Can you work these out from the model? Positions are in its coordinate system, mm. A direction names the side the tool comes from. Give positions to 0.01 mm unless a question says otherwise; leave off trailing zeros. Loops run counter-clockwise (first coordinate to the right, second up) from the corner with the lowest first, then second, coordinate; pieces in that order, holes last. Notation, with made-up numbers: M 5.25,52 L 22.25,52 A35 ccw 22.25,86 Z; hole C -32.5,21 d1. An arc over 180 degrees is marked long. Answer as a JSON object with one key per item and string values.
```python
from build123d import *

# Parameters (mm, degrees)
BOSS_EXTRUDE1_DEPTH  = 49
SKETCH2_R            = 2.5
CUT_EXTRUDE1_DEPTH   = 8.5
SKETCH4_W            = 79
SKETCH4_H            = 39.5
BOSS_EXTRUDE2_DEPTH  = 6
BOSS_EXTRUDE3_DEPTH  = 4
SKETCH5_R            = 2
CUT_EXTRUDE3_DEPTH   = 10
BOSS_EXTRUDE4_DEPTH  = 4
SKETCH8_R            = 1.5
CUT_EXTRUDE4_DEPTH   = 8
FILLET1_R            = 6
FILLET2_R            = 5
CUT_EXTRUDE5_DEPTH   = 3
CUT_EXTRUDE6_DEPTH   = 50
FILLET3_R            = 4
CUT_EXTRUDE7_DEPTH   = 3
LPATTERN1_COUNT      = 2
LPATTERN1_PITCH      = 67
LPATTERN1_COUNT_DIR2 = 2
LPATTERN1_PITCH_DIR2 = 27.5


with BuildPart() as part:
    # Sketch1 → Boss-Extrude1 (new body)
    with BuildSketch(Plane.XY):
        Polygon((4, 7.5), (4, 19.5), (0, 19.5), (0, 0), (55, 0), (55, 7.5), align=None)
    extrude(amount=BOSS_EXTRUDE1_DEPTH)

    # Sketch2 → Cut-Extrude1 (cut, through all)
    with BuildSketch(Plane(origin=(0, 7.5, 0), x_dir=(1, 0, 0), z_dir=(0, 1, 0))):
        with Locations(Location((12, -12.5, 0), (0, 0, 270))):  # turned: the seam where the file's is
            Circle(SKETCH2_R)
        with Locations(Location((43, -12.5, 0), (0, 0, 270))):  # turned: the seam where the file's is
            Circle(SKETCH2_R)
        with Locations(Location((12, -43.5, 0), (0, 0, 270))):  # turned: the seam where the file's is
            Circle(SKETCH2_R)
        with Locations(Location((43, -43.5, 0), (0, 0, 270))):  # turned: the seam where the file's is
            Circle(SKETCH2_R)
        with BuildLine():
            Line((14.460001345, -31.494057109), (19.150704606, -49))
            Line((19.150704606, -49), (35.849295394, -49))
            Line((35.849295394, -49), (40.539998655, -31.494057109))
            ThreePointArc((40.539998655, -31.494057109), (27.5, -14.5), (14.460001345, -31.494057109))
        make_face()
    extrude(amount=-CUT_EXTRUDE1_DEPTH, mode=Mode.SUBTRACT)

    # Sketch4 → Boss-Extrude2 (add)
    with BuildSketch(Plane(origin=(0, 0, 0), x_dir=(-1, 0, 0), z_dir=(0, 0, -1))):
        with Locations((-27.5, -0.25)):
            Rectangle(SKETCH4_W, SKETCH4_H)
    extrude(amount=-BOSS_EXTRUDE2_DEPTH)

    # Sketch6 → Boss-Extrude3 (add)
    with BuildSketch(Plane.ZY):
        Polygon((6, -20), (49, 0), (6, 0), align=None)
    extrude(amount=-BOSS_EXTRUDE3_DEPTH)

    # Sketch5 → Cut-Extrude3 (cut)
    with BuildSketch(Plane(origin=(0, 0, 0), x_dir=(-1, 0, 0), z_dir=(0, 0, -1))):
        with Locations((-61, 13.5)):
            Circle(SKETCH5_R)
        with Locations((-61, -14)):
            Circle(SKETCH5_R)
        with Locations((6, 13.5)):
            Circle(SKETCH5_R)
        with Locations((6, -14)):
            Circle(SKETCH5_R)
    extrude(amount=-CUT_EXTRUDE3_DEPTH, mode=Mode.SUBTRACT)

    # Sketch7 → Boss-Extrude4 (add)
    with BuildSketch(Plane(origin=(55, 0, 0), x_dir=(0, 0, -1), z_dir=(1, 0, 0))):
        Polygon((-49, 7.5), (-6, 19.5), (0, 19.5), (0, -20), (-6, -20), (-49, 0), align=None)
    extrude(amount=-BOSS_EXTRUDE4_DEPTH)

    # Sketch8 → Cut-Extrude4 (cut)
    with BuildSketch(Plane.ZY):
        with Locations(Location((43, 13, 0), (0, 0, 270))):  # turned: the seam where the file's is
            Circle(SKETCH8_R)
        with Locations(Location((43, 3.5, 0), (0, 0, 270))):  # turned: the seam where the file's is
            Circle(SKETCH8_R)
    extrude(amount=-CUT_EXTRUDE4_DEPTH, mode=Mode.SUBTRACT)

    # Fillet1
    fillet1_edges = [part.edges().sort_by_distance(p)[0] for p in [
        (67, 19.5, 3),
        (-12, 19.5, 3),
        (-12, -20, 3),
        (67, -20, 3),
    ]]
    fillet(fillet1_edges, radius=FILLET1_R)

    # Fillet2
    fillet2_edges = [part.edges().sort_by_distance(p)[0] for p in [
        (35.849295394, 3.75, 49),
        (19.150704606, 3.75, 49),
    ]]
    fillet(fillet2_edges, radius=FILLET2_R)

    # Sketch9 → Cut-Extrude5 (cut)
    with BuildSketch(Plane.XY.offset(6)):
        Polygon((-6, 16.790896534), (-8.85, 15.145448267), (-8.85, 11.854551733), (-6, 10.209103466), (-3.15, 11.854551733), (-3.15, 15.145448267), align=None)
        Polygon((-6, -10.709103466), (-8.85, -12.354551733), (-8.85, -15.645448267), (-6, -17.290896534), (-3.15, -15.645448267), (-3.15, -12.354551733), align=None)
        Polygon((61, -10.709103466), (58.15, -12.354551733), (58.15, -15.645448267), (61, -17.290896534), (63.85, -15.645448267), (63.85, -12.354551733), align=None)
        Polygon((61, 10.209103466), (63.85, 11.854551733), (63.85, 15.145448267), (61, 16.790896534), (58.15, 15.145448267), (58.15, 11.854551733), align=None)
    extrude(amount=-CUT_EXTRUDE5_DEPTH, mode=Mode.SUBTRACT)

    # Sketch10 → Cut-Extrude6 (cut, through all)
    with BuildSketch(Plane(origin=(0, 0, 0), x_dir=(-1, 0, 0), z_dir=(0, 0, -1))):
        with BuildLine():
            Line((-61, 19.5), (-61, 26.194717678))
            Line((-61, 26.194717678), (-93.21372943, 26.194717678))
            Line((-93.21372943, 26.194717678), (-93.21372943, -32.483465835))
            Line((-93.21372943, -32.483465835), (20.656804912, -32.483465835))
            Line((20.656804912, -32.483465835), (20.656804912, 27.240467483))
            Line((20.656804912, 27.240467483), (6, 27.240467483))
            Line((6, 27.240467483), (6, 19.5))
            ThreePointArc((6, 19.5), (10.987484336, 16.835416016), (11.545111711, 11.208333333))
            ThreePointArc((11.545111711, 11.208333333), (9.270670267, -0.25), (11.545111711, -11.708333333))
            ThreePointArc((11.545111711, -11.708333333), (10.460015748, -18.013509627), (4.303797468, -19.755249514))
            ThreePointArc((4.303797468, -19.755249514), (-27.5, -15.166177907), (-59.303797468, -19.755249514))
            ThreePointArc((-59.303797468, -19.755249514), (-65.460015748, -18.013509627), (-66.545111711, -11.708333333))
            ThreePointArc((-66.545111711, -11.708333333), (-64.270670267, -0.25), (-66.545111711, 11.208333333))
            ThreePointArc((-66.545111711, 11.208333333), (-65.987484336, 16.835416016), (-61, 19.5))
        make_face()
    extrude(amount=-CUT_EXTRUDE6_DEPTH, mode=Mode.SUBTRACT)

    # Fillet3
    fillet3_edges = [part.edges().sort_by_distance(p)[0] for p in [
        (2, 19.5, 49),
    ]]
    fillet(fillet3_edges, radius=FILLET3_R)

    # Sketch11 → Cut-Extrude7 (cut)
    with BuildSketch(Plane.XY.offset(6)):
        with BuildLine():
            ThreePointArc((-9.35, 15.434123402), (-8.85, 13.5), (-9.35, 11.565876598))
            ThreePointArc((-9.35, 11.565876598), (-7.425, 11.031827599), (-6, 9.631753196))
            ThreePointArc((-6, 9.631753196), (-4.575, 11.031827599), (-2.65, 11.565876598))
            ThreePointArc((-2.65, 11.565876598), (-3.15, 13.5), (-2.65, 15.434123402))
            ThreePointArc((-2.65, 15.434123402), (-4.575, 15.968172401), (-6, 17.368246804))
            ThreePointArc((-6, 17.368246804), (-7.425, 15.968172401), (-9.35, 15.434123402))
        make_face()
    cut_extrude7 = extrude(amount=-CUT_EXTRUDE7_DEPTH, mode=Mode.SUBTRACT)

    # LPattern1: Cut-Extrude7 2 × 2
    with Locations(*[(i * LPATTERN1_PITCH, -j * LPATTERN1_PITCH_DIR2, 0) for i in range(LPATTERN1_COUNT) for j in range(LPATTERN1_COUNT_DIR2) if (i, j) != (0, 0)]):
        add(cut_extrude7, mode=Mode.SUBTRACT)


solid = part.part
```
1) If we mould it in two halves opening along Z, with no side actions, what happens to faces 1 (the flat face through (28, 0, 0)), 2 (the cylindrical face through (1.972, 13.325, 41.536)), 3 (the flat face through (39.017, 3.802, 37.178)), 4 (the cylindrical face through (62.474, 14.852, 1.479))? For each: +Z half, -Z half, draft (parallel to the pull), parting line (faces both ways), or undercut.
Answer list:
{"face 1": "-Z half", "face 2": "undercut", "face 3": "undercut", "face 4": "draft"}
2) Suppose I cut it at B-B, the plane y = 3. Write out the boundary of the cut face in (x, z).
Answer list:
{"outline": "M -9.45,0 L 64.45,0 L 64.45,6 L 55,6 L 55,49 L 42.37,49 A5 ccw 37.54,42.71 L 40.54,31.49 A13.5 cw long 14.46,31.49 L 17.46,42.71 A5 ccw 12.63,49 L 0,49 L 0,44.41 L 8,44.41 L 8,41.59 L 0,41.59 L 0,6 L -9.45,6 Z; hole C 12,12.5 d5; hole C 12,43.5 d5; hole C 43,12.5 d5; hole C 43,43.5 d5"}
3) For faces 5 (the flat face through (4, -7, 22)), 6 (the flat face through (61, 16, 3)), 7 (the flat face through (53.028, 13.416, 27.801)), which set-ups out of +Z, -Z, +X, -X, +Y, -Y let a thin tool reach every point of the face, with its end or its side?
Answer list:
{"face 5": "+Z, -Y", "face 6": "+Z", "face 7": "+Z, +X, +Y"}
4) Suppose I cut it at A-A, the plane z = 12.5. Write out the boundary of the cut face in (x, y), and give its area (3 significant figures).
Answer list:
{"outline": "M 0,-16.98 L 4,-16.98 L 4,0 L 9.5,0 L 9.5,7.5 L 4,7.5 L 4,19.5 L 0,19.5 Z; M 14.5,0 L 40.5,0 L 40.5,7.5 L 14.5,7.5 Z; M 45.5,0 L 51,0 L 51,-16.98 L 55,-16.98 L 55,17.69 L 51,17.69 L 51,7.5 L 45.5,7.5 Z", "area": "562 mm^2"}
5) Suppose I cut it at C-C, the plane y = -3. Write out the boundary of the cut face in (x, z).
Answer list:
{"outline": "M -9.4,0 L 64.4,0 L 64.4,6 L 55,6 L 55,42.55 L 51,42.55 L 51,6 L 4,6 L 4,42.55 L 0,42.55 L 0,6 L -9.4,6 Z"}
6) Suppose I cut it at D-D, the plane x = 31.5. Write out the boundary of the cut face in (y, z), and give its area (3 significant figures).
Answer list:
{"outline": "M -15.24,0 L 19.5,0 L 19.5,6 L 7.5,6 L 7.5,15.11 L 0,15.11 L 0,6 L -15.24,6 Z", "area": "277 mm^2"}
7) Will these pins go through, and if not, where does the flat tip stop? pin 1 Ø8 at (x, z) = (43.5, 40) entering from +Y; pin 2 Ø4 at (x, y) = (9, 10) entering from +Z; pin 3 Ø3.5 at (y, z) = (12.5, 27) entering from -X.
Answer list:
{"pin 1": "y = 7.5", "pin 2": "z = 6", "pin 3": "x = 0"}
8) Please list where these lines run through material, in increasing order: line 1 along Y through (x, z) = (-6, 2.25); line 2 along X through (y, z) = (-4, 21); line 3 along X through (y, z) = (3.5, 12.5). Write a range as from..to.
Answer list:
{"line 1": "-20..-16, -12..11.5, 15.5..19.5", "line 2": "0..4, 51..55", "line 3": "0..9.5, 14.5..40.5, 45.5..55"}
